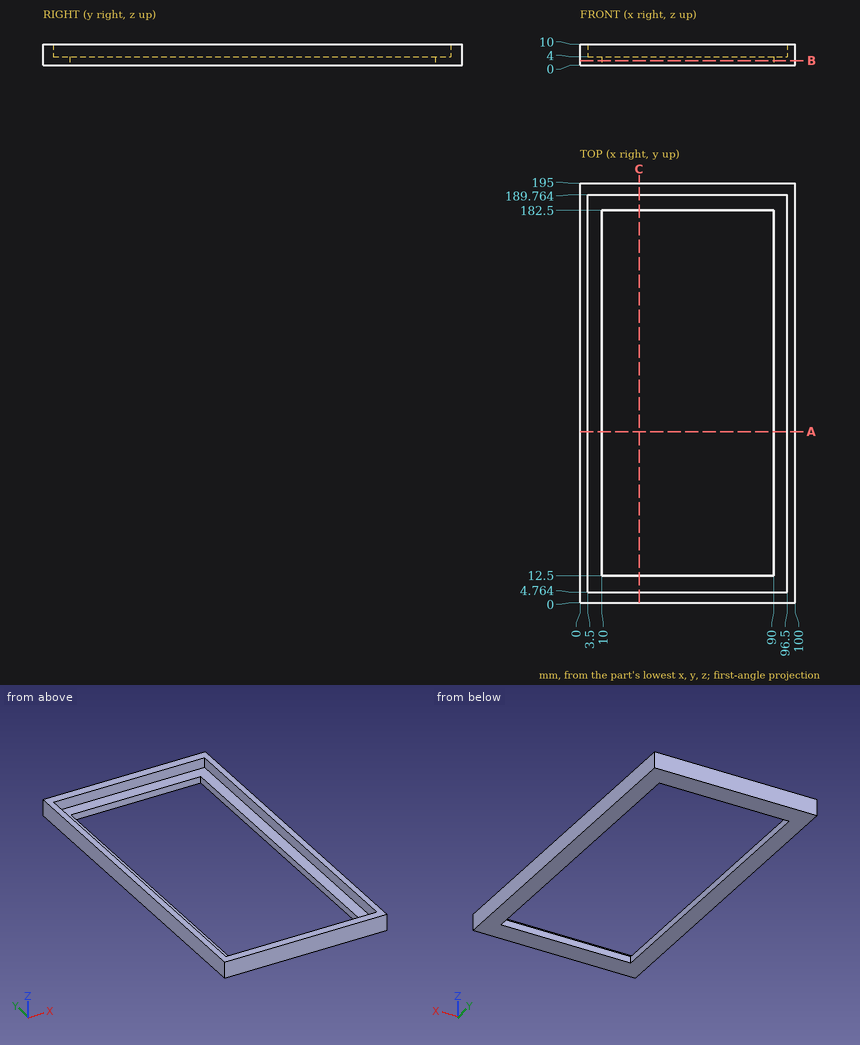
The figure shows three views and two pictorial views of one solid part (mm, origin at its lowest corner). Answer the questions. Round coordinates to 2 decimals unless told otherwise and drop trailing zeros. Write each loop counter-clockwise with the first axis right and the second up, starting at its lowest first coordinate (ties: lowest second). Pieces come first, ordered by that corner, then holes. Notation, with made-up numbers: (-39, -25.5) - (5, -25.5) arc R20 cw to (5, -16.5) - close; hole circle Ø10 at (3.5, -3.75). An arc over 180 degrees is marked (long way). One line per question, with ' | ' between items. Start each with the question number.
1. Find the intervals of material crossed by probe 1 along Y at (x, z) = (56, 8.5); probe 2 along Y at (x, z) = (53, 1.25); probe 3 along X at (y, z) = (88, 2.75), in increasing order. Write a range as [from, to].
2. This flat-tipped pin is pushed along its axis until it touches: pin 1 (8 mm diameter, centred on x = 85.5, y = 152, fed in from +Z). Where does it stop, or does it pass through?
3. Section A-A (y = 79.5) is taken. Determine the outline of the cut face in (x, z), and give its area (3 significant figures).
4. Section B-B (z = 2.25) is taken. Determine the outline of the cut face in (x, y), and give its area (3 significant figures).
5. Section C-C (x = 27.5) is taken. Determine the outline of the cut face in (y, z).
Filled in:
1) probe 1: [0, 4.76], [189.76, 195] | probe 2: [0, 12.5], [182.5, 195] | probe 3: [0, 10], [90, 100]
2) pin 1: through
3) outline: (0, 0) - (10, 0) - (10, 4) - (3.5, 4) - (3.5, 10) - (0, 10) - close; (90, 0) - (100, 0) - (100, 10) - (96.5, 10) - (96.5, 4) - (90, 4) - close | area: 122 mm²
4) outline: (0, 0) - (100, 0) - (100, 195) - (0, 195) - close; hole (10, 12.5) - (90, 12.5) - (90, 182.5) - (10, 182.5) - close | area: 5,900 mm²
5) outline: (0, 0) - (12.5, 0) - (12.5, 4) - (4.76, 4) - (4.76, 10) - (0, 10) - close; (182.5, 0) - (195, 0) - (195, 10) - (189.76, 10) - (189.76, 4) - (182.5, 4) - close
